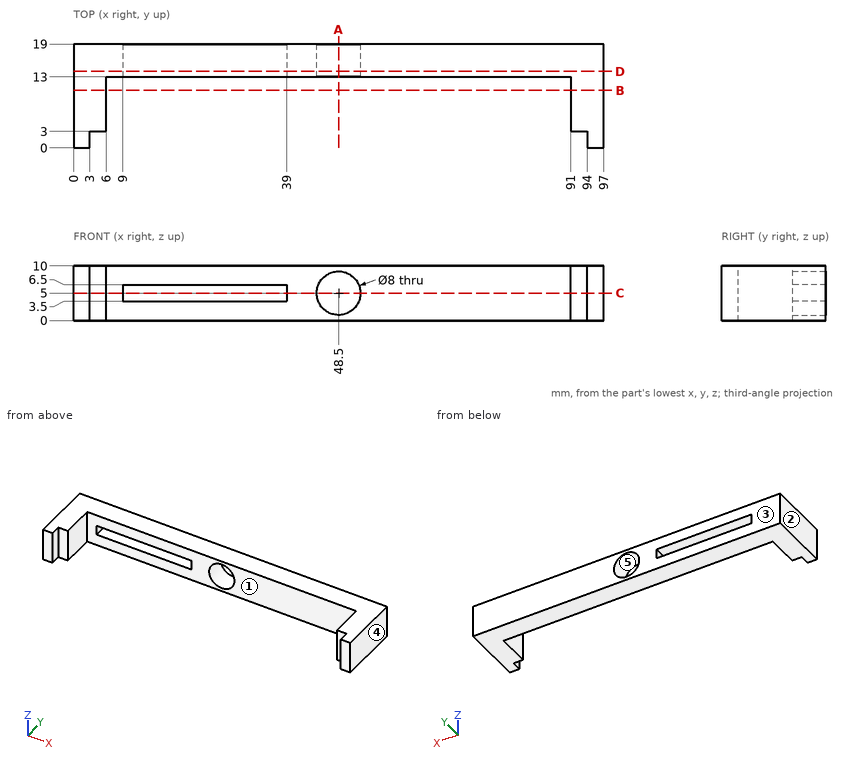
Answer from the drawing. Dimensions are ordinates in mm from the lowest x, y and z of the part. A direction names the side the tool comes from. Round coordinates to 2 decimals unless told otherwise and drop trailing zeros. Loops run counter-clockwise (first coordinate to the right, second up) from the corner with the lowest first, then second, coordinate; pieces in that order, holes last. Notation, with made-up numbers: (63.25, 45) - (109.25, 45) arc R28 ccw to (109.25, 70) - close; hole circle Ø7 at (-16, -14.5). An arc over 180 degrees is marked (long way). Return JSON: item names as keys, results as strings. Group by question number.
1. Each of these flat-tipped pins is pushed along its axis until it touches: P1, Ø0.9, axis at x = 93, z = 6, coming from the -Y side; P2, Ø5, axis at x = 43, z = 6.5, coming from the -Y side; P3, Ø1, axis at x = 33, z = 5.5, coming from the +Y side. Where does it stop, or does it pass through?
2. Which of the six approach directions +Z, -Z, +X, -X, +Y, -Y give full straight-line access (tool end or side, diameter ignored) to the marked faces 1 and 2?
3. The part is cut by section D-D on y = 14. Determine the outline of the cut face in (x, z), then the cut area to 3 significant figures.
4. The part is cut by section C-C on z = 5. Determine the outline of the cut face in (x, y), then the cut area to 3 significant figures.
5. The part is cut by section A-A on x = 48.5. Determine the outline of the cut face in (y, z).
6. Consider probe 1 along X at (y, z) = (15.95, 5); probe 2 along Z at (x, y) = (48.5, 17.25); probe 3 along Z at (x, y) = (19, 16). Determine where each line is inside the solid, lowest interval first.
7. The mould has two halves that part along X. Classify the marked faces 3, 4 and 5: pulls with the +X half, pulls with the -X half, needs draft (parallel to the pull), parting line crosses it, or undercut.
8. The part is cut by section B-B on y = 10.5. Determine the outline of the cut face in (x, z).
Resolved:
{
 "1": {"P1": "stops at y = 3", "P2": "stops at y = 13", "P3": "passes through"},
 "2": {"face 1": "+Z, -Z, -Y", "face 2": "+Z, -Z, -X, +Y, -Y"},
 "3": {"outline": "(0, 0) - (97, 0) - (97, 10) - (0, 10) - close; hole (9, 3.5) - (39, 3.5) - (39, 6.5) - (9, 6.5) - close; hole circle Ø8 at (48.5, 5)", "area": "830 mm²"},
 "4": {"outline": "(0, 0) - (3, 0) - (3, 3) - (6, 3) - (6, 13) - (9, 13) - (9, 19) - (0, 19) - close; (39, 13) - (44.5, 13) - (44.5, 19) - (39, 19) - close; (52.5, 13) - (91, 13) - (91, 3) - (94, 3) - (94, 0) - (97, 0) - (97, 19) - (52.5, 19) - close", "area": "492 mm²"},
 "5": {"outline": "(13, 0) - (19, 0) - (19, 1) - (13, 1) - close; (13, 9) - (19, 9) - (19, 10) - (13, 10) - close"},
 "6": {"probe 1": "x = 0 to 9, 39 to 44.5, 52.5 to 97", "probe 2": "z = 0 to 1, 9 to 10", "probe 3": "z = 0 to 3.5, 6.5 to 10"},
 "7": {"face 3": "needs draft", "face 4": "pulls with the +X half", "face 5": "undercut"},
 "8": {"outline": "(0, 0) - (6, 0) - (6, 10) - (0, 10) - close; (91, 0) - (97, 0) - (97, 10) - (91, 10) - close"}
}
